Input: part model. Units: mm. Frame: model coordinates. A direction names the side the tool comes from. Round coordinates to 2 decimals unless told otherwise and drop trailing zeros. Order: outer loops, then holes, each group sorted by start corner. A loop starts at its lowest first (then second) coordinate and runs counter-clockwise, first axis right, second up. Notation, with made-up numbers: (-10.5, -40) -> (1.5, -40) arc R20 ccw to (1.5, -12) -> close; hole circle Ø1 at (-37.5, 3.25). An arc over 180 degrees is marked (long way). Answer as CSV lines item,"result". Start each with the question number.
1) Section query D-D, the plane z = 614.5. Output: boundary loops of the cut face in (x, y) (3 decimals).
2) First-contact query: P1, Ø4, axis at x = 16.5, y = 44, coming from the -Z side; P2, Ø5.5, axis at x = -21.04, z = 663.49, coming from the -Y side; P3, Ø1, axis at x = 26, y = 45.5, coming from the +Z side. Flat tips, straight axial feed; report the tip coordinate or a pass-through.
3) Access query for faces 1 (the face through (23.15, 41.42, 674.11)), 2 (the face through (0, 34, 601.578)), 3 (the face through (1, 40.009, 584)). Directions: +Z, -Z, +X, -X, +Y, -Y. A direction counts if a zero-diameter tool reaches every point of the face in a straight line with its end or side. Return the directions, or none.
4) Section query A-A, the plane z = 674. Output: boundary loops of the cut face in (x, y) (3 decimals).
5) Section query B-B, the plane y = 46.25. Output: boundary loops of the cut face in (x, z) (1 decimal).
6) Section query C-C, the plane x = -12. Output: boundary loops of the cut face in (y, z), and give its area (3 significant figures).
7) Line query: L1, parallel to Z at x = 9.5, y = 33; L2, parallel to Z at x = -19, y = 43.75; L3, parallel to X at y = 47.25, z = 607.5. Output: solid intervals per line, ascending.
Autodesk Inventor part; units mm, degrees
ref_plane "Work Plane1" through (0, 0, 482.6) normal (1, 0, 0) x (0, 1, 0)
ref_plane "YZ Plane" through (0, 0, 0) normal (1, 0, 0) x (0, 1, 0)
ref_plane "XZ Plane" through (0, 0, 0) normal (0, 1, 0) x (-1, 0, 0)
sketch "Sketch1" plane through (0, 0, 0) normal (0, 1, 0) x (-1, 0, 0)
  line L0 (-40, 482.6) -> (-40, -482.6)
  line L1 (-40, -482.6) -> (40, -482.6)
  line L2 (40, -482.6) -> (40, 482.6)
  line L3 (40, 482.6) -> (-40, 482.6)
  line L4 (-40, 482.6) -> (40, -482.6) construction
  line L5 (-40, -482.6) -> (40, 482.6) construction
  point P0 (0, 0)
  dimension "d0" = 965.2
  dimension "d1" = 80
extrude "Extrusion1" add sketch "Sketch1" against normal blind 15.5448
ref_plane "Work Plane1" through (0, 0, 482.6) normal (1, 0, 0) x (0, 1, 0)
sketch "Sketch2" plane through (0, 0, 482.6) normal (1, 0, 0) x (0, 1, 0)
  line L0 (0, -965.2) -> (0, 0)
  line L1 (0, -965.2) -> (-15.5448, -965.2)
  line L2 (-15.5448, 0) -> (-15.5448, -965.2)
  line L3 (0, 0) -> (-15.5448, 0)
  line L4 (41.9902, -1050.1493) -> (41.9902, -1135.1493)
  line L5 (57.0671, -1050.1493) -> (57.0671, -1135.1493)
  line L6 (57.0671, -1135.1493) -> (41.9902, -1135.1493)
  line L7 (41.9902, -1092.6493) -> (57.0671, -1092.6493) construction
  line L8 (-15.5448, 0) -> (-15.5448, -965.2) construction
  line L9 (-15.5448, -965.2) -> (-15.5448, -1004.6981) construction
  line L10 (-15.5448, -1004.6981) -> (41.9902, -1021.6042) construction
  line L11 (41.9902, -1021.6042) -> (41.9902, -1050.1493) construction
  spline S0 degree 3 poles (-15.5448, -965.2) (-15.5448, -1004.6981) (41.9902, -1021.6042) (41.9902, -1050.1493) knots 1 1 1 1 2 2 2 2
  line L12 (57.0671, -1050.1493) -> (57.0671, -1021.6042) construction
  line L13 (57.0671, -1021.6042) -> (0, -1003.1803) construction
  line L14 (0, -965.2) -> (0, 0) construction
  line L15 (0, -1003.1803) -> (0, -965.2) construction
  spline S1 degree 3 poles (57.0671, -1050.1493) (57.0671, -1021.6042) (0, -1003.1803) (0, -965.2) knots 1 1 1 1 2 2 2 2
  point P0 (0, -482.6)
  dimension "d4" = 85
  dimension "d5" = 15.0769
sketch "Sketch3" plane through (0, 0, 482.6) normal (1, 0, 0) x (0, 1, 0)
  line L0 (0, 0) -> (0, -965.2)
  line L1 (0, 0) -> (-15.5448, 0)
  line L2 (-15.5448, -965.2) -> (-15.5448, 0)
  line L3 (0, -965.2) -> (-15.5448, -965.2)
  arc A0 (2.1293, 48.5593) -> (-15.5448, 0) centre (60, 0) ccw
  arc A1 (14.0373, 38.5673) -> (0, 0) centre (60, 0) ccw
  line L4 (2.1293, 48.5593) -> (18.199, 67.7104)
  line L5 (0, 0) -> (-15.5448, 0) construction
  line L6 (2.1293, 48.5593) -> (14.0373, 38.5673) construction
  line L7 (14.0373, 38.5673) -> (30.107, 57.7184)
  arc A2 (18.199, 67.7104) -> (32.2363, 106.2776) centre (-27.7637, 106.2776) ccw
  arc A3 (30.107, 57.7184) -> (47.7811, 106.2776) centre (-27.7637, 106.2776) ccw
  line L8 (32.2363, 106.2776) -> (32.2363, 233.2776)
  line L9 (32.2363, 233.2776) -> (47.7811, 233.2776)
  line L10 (47.7811, 233.2776) -> (47.7811, 106.2776)
  line L11 (30.107, 57.7184) -> (18.199, 67.7104) construction
  line L12 (32.2363, 106.2776) -> (47.7811, 106.2776) construction
  point P0 (0, -482.6)
  dimension "d17" = 127
  dimension "d18" = 140
  dimension "d19" = 60
  dimension "d21" = 140
  dimension "d22" = 25
extrude "Extrusion2" add sketch "Sketch3" along normal up to surface (80 mm away) from surface at -40 contours L1 A0 L4 A2 L8 L9 L10 A3 L7 A1
sketch "Sketch9" plane through (-40, 47.7811, 588.8776) normal (0, 1, 0) x (1, 0, 0)
  line L0 (0, -127) -> (0, 0) construction
  line L1 (0, 0) -> (0, -127) construction
  line L2 (80, -127) -> (80, 0) construction
  line L3 (0, -127) -> (0, -49.1262)
  line L4 (80, 0) -> (80, -127)
  line L5 (80, -49.1262) -> (80, -127)
  arc A0 (0, -49.1262) -> (24.125, -127) centre (137.7482, -49.1262) ccw
  arc A1 (55.875, -127) -> (80, -49.1262) centre (-57.7482, -49.1262) ccw
  line L6 (24.125, -127) -> (55.875, -127)
  line L7 (0, -127) -> (80, -127)
  line L8 (55.875, -127) -> (80, -127)
  line L9 (80, -127) -> (80, -49.1262)
  line L10 (0, -127) -> (24.125, -127)
  line L11 (55.875, -127) -> (80, -127)
  line L12 (24.125, -127) -> (0, -127)
  point P0 (40, 588.8776)
  dimension "d41" = 31.75
sketch "Sketch10" plane through (-40, 47.7811, 588.8776) normal (0, 1, 0) x (1, 0, 0)
  line L0 (11.425, -92.075) -> (68.575, -92.075) construction
  line L1 (68.575, -92.075) -> (68.575, -12.7) construction
  line L2 (68.575, -12.7) -> (11.425, -12.7) construction
  line L3 (11.425, -12.7) -> (11.425, -92.075) construction
  line L4 (11.425, -92.075) -> (68.575, -12.7) construction
  line L5 (68.575, -92.075) -> (11.425, -12.7) construction
  line L6 (12.6315, -90.043) -> (67.3685, -90.043)
  line L7 (67.3685, -90.043) -> (67.3685, -14.732)
  line L8 (67.3685, -14.732) -> (12.6315, -14.732)
  line L9 (12.6315, -14.732) -> (12.6315, -90.043)
  line L10 (12.6315, -90.043) -> (67.3685, -14.732) construction
  line L11 (67.3685, -90.043) -> (12.6315, -14.732) construction
  line L12 (18.965, -84.1375) -> (61.035, -84.1375) construction
  line L13 (61.035, -84.1375) -> (61.035, -20.6375) construction
  line L14 (61.035, -20.6375) -> (18.965, -20.6375) construction
  line L15 (18.965, -20.6375) -> (18.965, -84.1375) construction
  line L16 (18.965, -84.1375) -> (61.035, -20.6375) construction
  line L17 (61.035, -84.1375) -> (18.965, -20.6375) construction
  line L18 (18.965, -84.1375) -> (61.035, -84.1375) construction
  line L19 (61.035, -84.1375) -> (61.035, -74.6125) construction
  line L20 (61.035, -74.6125) -> (18.965, -74.6125) construction
  line L21 (18.965, -74.6125) -> (18.965, -84.1375) construction
  line L22 (68.575, -12.7) -> (80, -12.7) construction
  line L23 (11.425, -12.7) -> (0, -12.7) construction
  line L24 (0, -127) -> (0, 0) construction
  line L25 (80, -127) -> (80, 0)
  line L26 (0, 0) -> (80, 0)
  point P0 (40, 588.8776)
  point P1 (40, -52.3875)
  dimension "d33" = 57.15
  dimension "d34" = 79.375
  dimension "d35" = 54.737
  dimension "d36" = 75.311
  dimension "d37" = 42.07
  dimension "d38" = 63.5
  dimension "d39" = 9.525
  dimension "d40" = 12.7
extrude "Extrusion7" cut sketch "Sketch9" against normal through all
hole "Hole1" at (-21.035, 47.7811, 673.0151) at (-21.035, 47.7811, 663.4901) at (21.035, 47.7811, 673.0151) at (21.035, 47.7811, 663.4901) at (21.035, 47.7811, 609.5151) at (-21.035, 47.7811, 609.5151) direction (0, -1, 0) diameter 4.7625 end through all
sketch "Sketch11" plane through (-40, 32.2363, 588.8776) normal (0, -1, 0) x (1, 0, 0)
  line L0 (11.425, 92.075) -> (68.575, 92.075) construction
  line L1 (11.425, 12.7) -> (11.425, 92.075) construction
  line L2 (68.575, 92.075) -> (68.575, 12.7) construction
  line L3 (11.425, 12.7) -> (68.575, 12.7)
  line L4 (68.575, 12.7) -> (68.575, 92.075)
  line L5 (68.575, 92.075) -> (11.425, 92.075)
  line L6 (11.425, 92.075) -> (11.425, 12.7)
  line L7 (11.425, 12.7) -> (68.575, 92.075) construction
  line L8 (68.575, 12.7) -> (11.425, 92.075) construction
  point P0 (40, -588.8776)
  point P1 (40, 52.3875)
extrude "Extrusion8" cut sketch "Sketch11" against normal blind 3
sketch "Sketch12" plane through (-40, 47.7811, 588.8776) normal (0, 1, 0) x (1, 0, 0)
  line L0 (80, -127) -> (0, -127)
  line L1 (0, -127) -> (0, 0)
  line L2 (0, 0) -> (80, 0)
  line L3 (80, 0) -> (80, -127)
  line L4 (24.125, -127) -> (55.875, -127)
  line L5 (0, 0) -> (0, -49.1262)
  point P0 (40, 588.8776)
extrude "Extrusion9" cut sketch "Sketch12" against normal through all keep common part
sketch "Sketch13" plane through (40, 32.2363, 638.0038) normal (1, 0, 0) x (0, 0, -1)
  line L0 (49.1262, 15.5448) -> (49.1262, 0)
  line L1 (0, 15.5448) -> (49.1262, 15.5448)
  line L2 (0, 0) -> (0, 15.5448)
  line L3 (49.1262, 0) -> (0, 0)
  line L4 (26.1074, 3) -> (26.1074, 15.5448)
  line L5 (30.8699, 3) -> (30.8699, 15.5448)
  line L6 (-42.9488, 3) -> (36.4262, 3)
  line L7 (36.4262, 0) -> (36.4262, 3)
  line L8 (49.1262, 0) -> (59.1262, 0)
  line L9 (59.1262, 0) -> (59.1262, 7.7724)
  line L10 (59.1262, 7.7724) -> (49.1262, 7.7724)
  line L11 (49.1262, 7.7724) -> (49.1262, 0)
  line L12 (49.1262, 15.5448) -> (39.1262, 15.5448)
  line L13 (39.1262, 15.5448) -> (39.1262, 7.7724)
  line L14 (39.1262, 7.7724) -> (49.1262, 7.7724)
  line L15 (49.1262, 7.7724) -> (49.1262, 15.5448)
  line L16 (39.1262, 15.5448) -> (49.1262, 7.7724)
  line L17 (49.1262, 0) -> (49.1262, 15.5448)
  line L18 (39.1262, 15.5448) -> (49.1262, 15.5448)
  point P0 (638.0038, -32.2363)
  dimension "d58" = 10
extrude "Extrusion10" add sketch "Sketch13" against normal up to surface (80 mm away) contours L10 L9 L8 L0
properties part number "Metal Middle" material "Aluminum 6061"
Findings:
1,outline,"(-40, 32.236) -> (-28.575, 32.236) -> (-28.575, 35.236) -> (28.575, 35.236) -> (28.575, 32.236) -> (40, 32.236) -> (40, 47.781) -> (-40, 47.781) -> close"
2,P1,"stops at z = 588.88"
2,P2,"stops at y = 35.24"
2,P3,"stops at z = 699.52"
3,face 1,"+Y, -Y"
3,face 2,"-Y"
3,face 3,"-Z, +X, -X, +Y"
4,outline,"(-35.214, 32.236) -> (-28.575, 32.236) -> (-28.575, 35.236) -> (-23.203, 35.236) -> (-23.203, 47.781) -> (-35.214, 47.781) -> close; (-18.867, 35.236) -> (18.867, 35.236) -> (18.867, 47.781) -> (-18.867, 47.781) -> close; (23.203, 35.236) -> (28.575, 35.236) -> (28.575, 32.236) -> (35.214, 32.236) -> (35.214, 47.781) -> (23.203, 47.781) -> close"
5,outline,"(-40, 588.9) -> (40, 588.9) -> (40, 638) arc R137.7 ccw to (15.9, 715.9) -> (-15.9, 715.9) arc R137.7 ccw to (-40, 638) -> close; hole circle Ø4.8 at (-21, 609.5); hole circle Ø4.8 at (-21, 663.5); hole circle Ø4.8 at (-21, 673); hole circle Ø4.8 at (21, 609.5); hole circle Ø4.8 at (21, 663.5); hole circle Ø4.8 at (21, 673)"
6,outline,"(32.24, 578.88) -> (40.01, 578.88) -> (40.01, 588.88) -> (47.78, 588.88) -> (47.78, 715.88) -> (32.24, 715.88) -> (32.24, 680.95) -> (35.24, 680.95) -> (35.24, 601.58) -> (32.24, 601.58) -> close"
6,area,"1,810 mm^2"
7,L1,"z = 578.88 to 601.58, 680.95 to 715.88"
7,L2,"z = 588.88 to 608.28, 610.75 to 662.25, 664.73 to 671.78, 674.25 to 711.11"
7,L3,"x = -40 to -22.3, -19.77 to 19.77, 22.3 to 40"
